CAD build for the part. Positions are in the model's coordinates, mm. A direction names the side the tool comes from. Coordinates: 2 decimals unless noted, no trailing zeros. Loops run counter-clockwise (first coordinate to the right, second up) from the corner with the lowest first, then second, coordinate; pieces in that order, holes last.
1) Which spindle directions (+Z, -Z, +X, -X, +Y, -Y) get a long thin tool onto all of the face, cutting with end or side? Do faces 1 (the cylindrical face through (102.83, -21.76, -105.05)), 2 (the flat face through (1, -40, -19)), 3 (the flat face through (102, -40, -108)), 4 (the cylindrical face through (101.45, -1.48, -103.6)). Say none if no direction does.
2) Wall check: line 1 along Z through (x, y) = (14, -23); line 2 along Z through (x, y) = (126.5, -27.5); line 3 along X through (y, z) = (-33, -76.5). Give the ranges that are in metal, low to high.
3) Saw through at B-B, the plane y = -18. Write the cut outline in (x, z), and give its area (3 significant figures).
4) Saw through at A-A, the plane z = -30.5. Write the cut outline in (x, y).
5) Two-plate mould, pull along X, no slides. Class faces 5 (the flat face through (76, -23, 0)), 6 (the cylindrical face through (104.89, -19.72, -107.23)), 7 (the flat face through (3, -26, -74)): +X half, -X half, draft (parallel to the pull), parting line (faces both ways), or undercut.
6) Saw through at C-C, the plane x = 71.5. Write the cut outline in (y, z), and give its area (3 significant figures).
7) Pin check, flat tips, straight feed: pin 1 Ø1 at (y, z) = (-14.5, -41.5) entering from +X; pin 2 Ø1.5 at (y, z) = (-44.5, -2) entering from -X; pin 3 Ø3.5 at (x, y) = (98, -2) entering from -Z. Stop position of each tip, or through.
```python
from build123d import *

# Parameters (mm, degrees)
F1_DEPTH = 40
F2_W     = 3
F2_H     = 20
F2_W_2   = 20.007767
F2_H_2   = 3
F3_DEPTH = 20
F4_R     = 9.99
F5_R     = 9.99
F7_DEPTH = 40
F9_DEPTH = 37


with BuildPart() as f1:
    # F0 (on Front) → F1 (new body)
    with BuildSketch(Plane.XZ):
        with BuildLine():
            Line((0, 0), (0, -150))
            ThreePointArc((0, -150), (106.066017, -106.066017), (150, 0))
            Line((150, 0), (0, 0))
        make_face()
    extrude(amount=F1_DEPTH)

    # F2 (on face) → F3 (join)
    with BuildSketch(Plane.XZ.offset(40)):
        with Locations((1.5, -77.260775)):
            Rectangle(F2_W, F2_H)
        with Locations((77.210668, -1.5)):
            Rectangle(F2_W_2, F2_H_2)
    extrude(amount=F3_DEPTH)

    # F4
    f4_edges = [f1.edges().sort_by_distance(p)[0] for p in [
        (87.214552, -60, -1.5),
    ]]
    fillet(f4_edges, radius=F4_R)

    # F5
    f5_edges = [f1.edges().sort_by_distance(p)[0] for p in [
        (67.206785, -60, -1.5),
        (1.5, -60, -67.260775),
        (1.5, -60, -87.260775),
    ]]
    fillet(f5_edges, radius=F5_R)

    # F6 (on Front) → F7 (cut, through all)
    with BuildSketch(Plane.XZ):
        with BuildLine():
            Line((144.913773, -5), (5, -5))
            Line((5, -5), (5, -144.913773))
            ThreePointArc((5, -144.913773), (102.530487, -102.530487), (144.913773, -5))
        make_face()
    extrude(amount=F7_DEPTH, mode=Mode.SUBTRACT)

    # F8 (on face) → F9 (cut)
    with BuildSketch(Plane.XZ.offset(40)):
        with BuildLine():
            Line((146.969385, -3), (3, -3))
            Line((3, -3), (3, -146.969385))
            ThreePointArc((3, -146.969385), (103.944697, -103.944697), (146.969385, -3))
        make_face()
    extrude(amount=-F9_DEPTH, mode=Mode.SUBTRACT)


solid = f1.part
```
Data:
1. face 1: -Y
1. face 2: +Z, -X, -Y
1. face 3: -Z, +X, -Y
1. face 4: +Y, -Y
2. line 1: z = -149.35 to -146.33, -3 to 0
2. line 2: z = -80.61 to -74.88, -3 to 0
2. line 3: x = 0 to 3, 125.53 to 129.03
3. outline: (0, -150) arc R150 ccw to (150, 0) - (0, 0) - close; hole (3, -146.97) arc R147 ccw to (146.97, -3) - (3, -3) - close
3. area: 1,570 mm2
4. outline: (0, -40) - (3, -40) - (3, -3) - (5, -3) - (5, 0) - (0, 0) - close; (141.76, -3) - (143.8, -3) - (143.8, -40) - (146.87, -40) - (146.87, 0) - (141.76, 0) - close
5. face 5: draft
5. face 6: +X half
5. face 7: undercut
6. outline: (-58.22, -3) - (-3, -3) - (-3, -5) - (0, -5) - (0, 0) - (-58.22, 0) - close; (-40, -131.86) - (0, -131.86) - (0, -126.15) - (-3, -126.15) - (-3, -128.44) - (-40, -128.44) - close
6. area: 324 mm2
7. pin 1: stops at x = 144.29
7. pin 2: stops at x = 67.21
7. pin 3: stops at z = -115.05
